Verification items for the finished model (mm, model axes). A direction names the side the tool comes from. Give positions to 0.01 mm unless a question says otherwise; leave off trailing zeros. Order: outer loops, then holes, each group sorted by start corner. A loop starts at its lowest first (then second) coordinate and runs counter-clockwise, first axis right, second up. Notation, with made-up numbers: (23, 44.5) - (35, 44.5) arc R22 ccw to (35, 80.5) - close; hole circle Ø1 at (16.25, 1.5). An arc over 180 degrees is marked (long way). Answer as a JSON object with one key per item and string values. Group by question number.
(1) Section check A-A (z = 0). Record the boundary of the cut face in (x, y).
(2) Access from +Z, -Z, +X, -X, +Y, -Y to the whole of each face (thin tool, end or side, straight path). Record for faces 1 (the face through (-59.94, 134.93, -2.64)), 2 (the face through (30, 205, 2)), 3 (the face through (-163.252, 254.51, -75.357)), 4 (the face through (184.83, 294.93, 100.295)), 5 (the face through (0, 190, 1)).
(3) Section check B-B (x = 160). Record the boundary of the cut face in (y, z).
(4) Depth check by flat-ended pin: pin 1 Ø6 at (x, z) = (-96.5, 108) entering from -Y; pin 2 Ø1 at (x, y) = (-50, 192) entering from +Z; pin 3 Ø1 at (x, z) = (134.5, 111.5) entering from +Y; pin 4 Ø5 at (x, z) = (-125, 41.5) entering from +Y. Enter the tip coordinate at first touch or a pass-through.
(5) Section check D-D (z = -50). Record the boundary of the cut face in (x, y), then the cut area to 3 significant figures.
(6) Mould release check, pull along Z, two halves, no side actions. Record for faces 6 (the face through (-4.351, 74.23, -33.136)), 7 (the face through (-3, 175, 80)), 8 (the face through (79, 190, -110)), 9 (the face through (12, 290, 102)): +Z half, -Z half, draft (parallel to the pull), parting line (faces both ways), or undercut.
(7) Section check C-C (x = -47). Record the boundary of the cut face in (y, z), then the cut area to 3 significant figures.
(8) Thickness scan on line 1 (X direction, y = 259.5, z = -91.5); line 2 (Y direction, x = -9.5, z = -69.5); line 3 (X direction, y = 194.5, z = -72). Record the ranges inside material, lowest first.
```python
from build123d import *

# Parameters (mm, degrees)
SKETCH_3_R      = 60
EXTRUDE_1_DEPTH = 20
SKETCH_4_R      = 33.420656991
EXTRUDE_2_DEPTH = 110
SKETCH_7_R      = 60
EXTRUDE_4_DEPTH = 10
SKETCH_9_W      = 380
SKETCH_9_H      = 280
EXTRUDE_5_DEPTH = 20
SKETCH_11_W     = 380
SKETCH_11_H     = 60
EXTRUDE_6_DEPTH = 30
SKETCH_13_W     = 60
SKETCH_13_H     = 30
EXTRUDE_7_DEPTH = 280
SKETCH_14_R     = 15
EXTRUDE_8_DEPTH = 70
SKETCH_16_R     = 26.879561929
EXTRUDE_9_DEPTH = 10


with BuildPart() as part:
    # 草图3 → 凸台-拉伸1 (new body)
    with BuildSketch(Plane(origin=(0, 0, 0), x_dir=(1, 0, 0), z_dir=(0, 1, 0))):
        Circle(SKETCH_3_R)
    extrude(amount=EXTRUDE_1_DEPTH)

    # 草图4 → 凸台-拉伸2 (add)
    with BuildSketch(Plane(origin=(0, 20, 0), x_dir=(1, 0, 0), z_dir=(0, 1, 0))):
        Circle(SKETCH_4_R)
    extrude(amount=EXTRUDE_2_DEPTH)

    # 草图7 → 凸台-拉伸4 (add)
    with BuildSketch(Plane(origin=(0, 130, 0), x_dir=(1, 0, 0), z_dir=(0, 1, 0))):
        Circle(SKETCH_7_R)
    extrude(amount=EXTRUDE_4_DEPTH)

    # 草图9 → 凸台-拉伸5 (add)
    with BuildSketch(Plane(origin=(0, 140, 0), x_dir=(1, 0, 0), z_dir=(0, 1, 0))):
        Rectangle(SKETCH_9_W, SKETCH_9_H)
    extrude(amount=EXTRUDE_5_DEPTH)

    # 草图11 → 凸台-拉伸6 (add)
    with BuildSketch(Plane(origin=(0, 160, 0), x_dir=(1, 0, 0), z_dir=(0, 1, 0))):
        with Locations((0, 110)):
            Rectangle(SKETCH_11_W, SKETCH_11_H)
        with Locations((0, -110)):
            Rectangle(SKETCH_11_W, SKETCH_11_H)
    extrude(amount=EXTRUDE_6_DEPTH)

    # 草图13 → 凸台-拉伸7 (add)
    with BuildSketch(Plane.XY.offset(140)):
        with Locations((-160, 205)):
            Rectangle(SKETCH_13_W, SKETCH_13_H)
        with Locations((0, 205)):
            Rectangle(SKETCH_13_W, SKETCH_13_H)
        with Locations((160, 205)):
            Rectangle(SKETCH_13_W, SKETCH_13_H)
    extrude(amount=-EXTRUDE_7_DEPTH)

    # 草图14 → 凸台-拉伸8 (add)
    with BuildSketch(Plane(origin=(0, 220, 0), x_dir=(1, 0, 0), z_dir=(0, 1, 0))):
        with Locations((-160, 90)):
            Circle(SKETCH_14_R)
        with Locations((0, 90)):
            Circle(SKETCH_14_R)
        with Locations((160, 90)):
            Circle(SKETCH_14_R)
        with Locations((-160, -90)):
            Circle(SKETCH_14_R)
        with Locations((0, -90)):
            Circle(SKETCH_14_R)
        with Locations((160, -90)):
            Circle(SKETCH_14_R)
    extrude(amount=EXTRUDE_8_DEPTH)

    # 草图16 → 凸台-拉伸9 (add)
    with BuildSketch(Plane(origin=(0, 290, 0), x_dir=(1, 0, 0), z_dir=(0, 1, 0))):
        with Locations((-160, 90)):
            Circle(SKETCH_16_R)
        with Locations((0, 90)):
            Circle(SKETCH_16_R)
        with Locations((160, 90)):
            Circle(SKETCH_16_R)
        with Locations((-160, -90)):
            Circle(SKETCH_16_R)
        with Locations((0, -90)):
            Circle(SKETCH_16_R)
        with Locations((160, -90)):
            Circle(SKETCH_16_R)
    extrude(amount=EXTRUDE_9_DEPTH)


solid = part.part
```
Solutions:
{
 "1": {"outline": "(-190, 140) - (-60, 140) - (-60, 130) - (-33.42, 130) - (-33.42, 20) - (-60, 20) - (-60, 0) - (60, 0) - (60, 20) - (33.42, 20) - (33.42, 130) - (60, 130) - (60, 140) - (190, 140) - (190, 160) - (-190, 160) - close; (-190, 190) - (-130, 190) - (-130, 220) - (-190, 220) - close; (-30, 190) - (30, 190) - (30, 220) - (-30, 220) - close; (130, 190) - (190, 190) - (190, 220) - (130, 220) - close"},
 "2": {"face 1": "-Y", "face 2": "+Z, -Z, +Y", "face 3": "none", "face 4": "+Y", "face 5": "+X, -X"},
 "3": {"outline": "(140, -140) - (220, -140) - (220, -105) - (290, -105) - (290, -116.88) - (300, -116.88) - (300, -63.12) - (290, -63.12) - (290, -75) - (220, -75) - (220, 75) - (290, 75) - (290, 63.12) - (300, 63.12) - (300, 116.88) - (290, 116.88) - (290, 105) - (220, 105) - (220, 140) - (140, 140) - close; hole (160, -80) - (190, -80) - (190, 80) - (160, 80) - close"},
 "4": {"pin 1": "stops at y = 140", "pin 2": "passes through", "pin 3": "stops at y = 220", "pin 4": "stops at y = 160"},
 "5": {"outline": "(-190, 140) - (-33.17, 140) - (-33.17, 130) - (33.17, 130) - (33.17, 140) - (190, 140) - (190, 160) - (-190, 160) - close; (-190, 190) - (-130, 190) - (-130, 220) - (-190, 220) - close; (-33.17, 0) - (33.17, 0) - (33.17, 20) - (-33.17, 20) - close; (-30, 190) - (30, 190) - (30, 220) - (-30, 220) - close; (130, 190) - (190, 190) - (190, 220) - (130, 220) - close", "area": "15,000 mm2"},
 "6": {"face 6": "parting line", "face 7": "undercut", "face 8": "draft", "face 9": "undercut"},
 "7": {"outline": "(0, -37.3) - (20, -37.3) - (20, 37.3) - (0, 37.3) - close; (130, -37.3) - (140, -37.3) - (140, -140) - (190, -140) - (190, -80) - (160, -80) - (160, 80) - (190, 80) - (190, 140) - (140, 140) - (140, 37.3) - (130, 37.3) - close", "area": "11,400 mm2"},
 "8": {"line 1": "x = -174.92 to -145.08, -14.92 to 14.92, 145.08 to 174.92", "line 2": "y = 140 to 160, 190 to 220, 290 to 300", "line 3": "x = -190 to -130, -30 to 30, 130 to 190"}
}
